Here's the drawing with two shaded views (mm, measured from the low corner). I have some questions. Round coordinates to 2 decimals unless told otherwise and drop trailing zeros. Order: outer loops, then holes, each group sorted by start corner. A loop starts at its lowest first (then second) coordinate and runs counter-clockwise, first axis right, second up. Notation, with made-up numbers: M 82,-13 L 123,-13 A25 ccw 123,17 Z; hole C 57.25,-38.75 d5. An arc over 180 degrees is marked long. One line per question, with ' | ' between items.
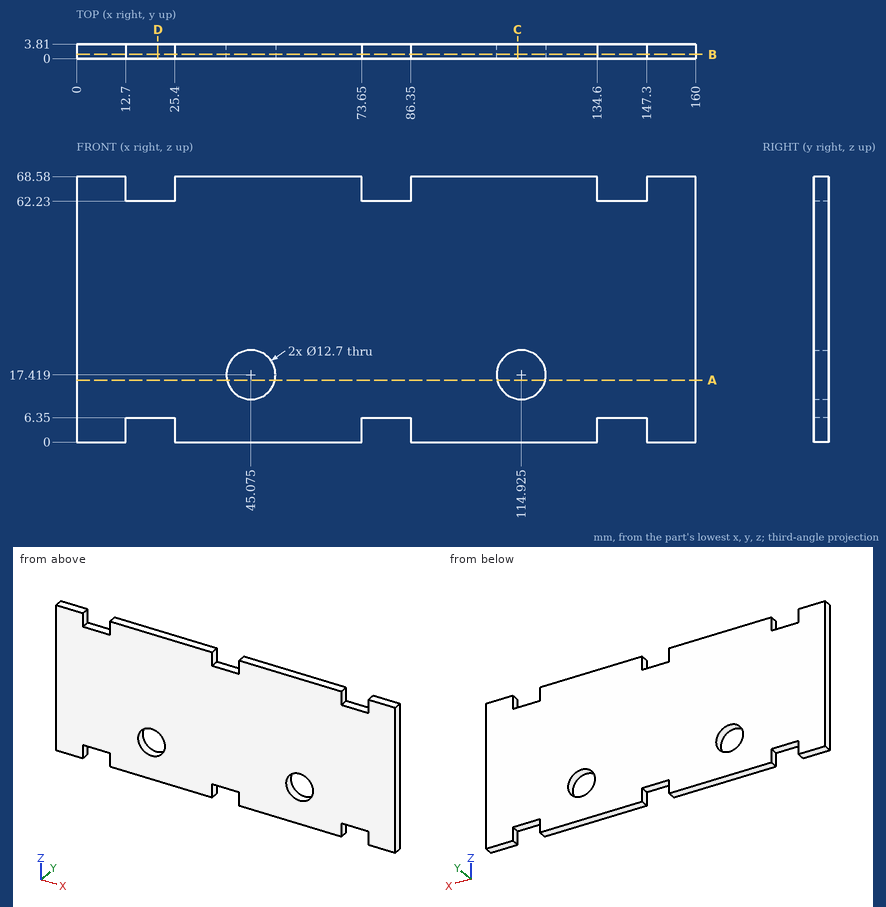
(1) If we section it at A-A on z = 16: Please give me the cut outline in (x, y) (1 decimal).
Final values:
outline: M 0,0 L 38.9,0 L 38.9,3.8 L 0,3.8 Z; M 51.3,0 L 108.7,0 L 108.7,3.8 L 51.3,3.8 Z; M 121.1,0 L 160,0 L 160,3.8 L 121.1,3.8 Z
(2) Will this pin go through, and if not, where does the flat tip stop? pin 1 Ø1.1 at (x, y) = (82, 1) entering from +Z.
Final values:
pin 1: z = 62.23
(3) If we section it at D-D on x = 21: Please give me the cut outline in (y, z).
Final values:
outline: M 0,6.35 L 3.81,6.35 L 3.81,62.23 L 0,62.23 Z
(4) Please list where these lines run through material, in increasing order: probe 1 along X at (y, z) = (0.5, 18); probe 2 along X at (y, z) = (1.75, 5); probe 3 along Z at (x, y) = (13.5, 0.45). Write a range as [from, to].
Final values:
probe 1: [0, 38.75], [51.4, 108.6], [121.25, 160] | probe 2: [0, 12.7], [25.4, 73.65], [86.35, 134.6], [147.3, 160] | probe 3: [6.35, 62.23]
(5) If we section it at C-C on x = 114: Please give me the cut outline in (y, z), plus the area to 3 significant figures.
Final values:
outline: M 0,0 L 3.81,0 L 3.81,11.14 L 0,11.14 Z; M 0,23.7 L 3.81,23.7 L 3.81,68.58 L 0,68.58 Z | area: 213 mm^2
(6) If we section it at B-B on y = 1.15: State how many separate pieces and enclosed holes the cut face has, plus the area to 3 significant figures.
Final values:
separate pieces: 1 | enclosed holes: 2 | area: 10,200 mm^2
